```python
from build123d import *

# Parameters (mm, degrees)
SKETCH1_R           = 4.015
SKETCH1_R_2         = 3.015
BOSS_EXTRUDE1_DEPTH = 1.85
SKETCH2_R           = 4.05
BOSS_EXTRUDE2_DEPTH = 0.6
SKETCH3_R           = 2.05
SKETCH3_R_2         = 1.05
BOSS_EXTRUDE3_DEPTH = 6


with BuildPart() as part:
    # Sketch1 → Boss-Extrude1 (new body)
    with BuildSketch(Plane(origin=(0, 0, 0), x_dir=(1, 0, 0), z_dir=(0, 1, 0))):
        Circle(SKETCH1_R)
        Circle(SKETCH1_R_2, mode=Mode.SUBTRACT)
    extrude(amount=BOSS_EXTRUDE1_DEPTH)

    # Sketch2 → Boss-Extrude2 (add)
    with BuildSketch(Plane(origin=(0, 0, 0), x_dir=(1, 0, 0), z_dir=(0, 1, 0))):
        Circle(SKETCH2_R)
    extrude(amount=-BOSS_EXTRUDE2_DEPTH)

    # Sketch3 → Boss-Extrude3 (add)
    with BuildSketch(Plane.XZ.offset(0.6)):
        Circle(SKETCH3_R)
        Circle(SKETCH3_R_2, mode=Mode.SUBTRACT)
    extrude(amount=BOSS_EXTRUDE3_DEPTH)


solid = part.part
```
Here's how the part is built. I have some questions about the finished solid (model axes, mm). A direction names the side the tool comes from. Give positions to 0.01 mm unless a question says otherwise; leave off trailing zeros. Loops run counter-clockwise (first coordinate to the right, second up) from the corner with the lowest first, then second, coordinate; pieces in that order, holes last. Notation, with made-up numbers: M 83.25,84.5 L 114.25,84.5 A34 ccw 114.25,120.5 Z; hole C 38,25.5 d6. An arc over 180 degrees is marked long. Put each result on its own line as item: value. Start each with the question number.
(1) I want a section at C-C on y = 0.75. Please give me the cut outline in (x, z) (3 decimals), then the cut area to 3 significant figures.
(2) I need wall thicknesses on line 1 along Z through (x, y) = (0, 0.9) (3 decimals); line 2 along Z through (x, y) = (0, -2.25); line 3 along Y through (x, z) = (-1.5, 3.5). Which ranges of each line are inside material? Lowest first, please. Write a range as [from, to].
(3) I want a section at A-A on z = 0. Please give me the cut outline in (x, y) (3 decimals), then the cut area to 3 significant figures.
(4) Will these pins go through, and if not, where does the flat tip stop? pin 1 Ø3 at (x, z) = (1, -0.5) entering from +Y; pin 2 Ø1 at (x, z) = (3, -2.5) entering from -Y; pin 3 Ø3 at (x, y) = (-3, -5) entering from -Z; pin 4 Ø2.5 at (x, z) = (1, 0) entering from -Y.
(5) For faces 1 (the cylindrical face through (-0.654, 0.912, 2.943)), 2 (the flat face through (1, -6.6, -1)), 3 (the flat face through (-2, -0.6, -1)), which set-ups out of +Z, -Z, +X, -X, +Y, -Y let a thin tool reach every point of the face, with its end or its side?
(6) I want a section at B-B on x = 0. Please give me the cut outline in (y, z) (3 decimals).
(7) If we mould it in two halves opening along Z, with no side actions, what happens to faces 4 (the flat face through (-3, 1.85, -2)), 5 (the cylindrical face through (-0.878, -0.296, 3.954)), 6 (the flat face through (0, -0.6, 0))? For each: +Z half, -Z half, draft (parallel to the pull), parting line (faces both ways), or undercut.
Answer block:
1. outline: C 0,0 d8.03; hole C 0,0 d6.03
1. area: 22.1 mm^2
2. line 1: [-4.015, -3.015], [3.015, 4.015]
2. line 2: [-2.05, -1.05], [1.05, 2.05]
2. line 3: [-0.6, 1.85]
3. outline: M -4.05,-0.6 L -2.05,-0.6 L -2.05,-6.6 L -1.05,-6.6 L -1.05,-0.6 L 1.05,-0.6 L 1.05,-6.6 L 2.05,-6.6 L 2.05,-0.6 L 4.05,-0.6 L 4.05,0 L 4.015,0 L 4.015,1.85 L 3.015,1.85 L 3.015,0 L -3.015,0 L -3.015,1.85 L -4.015,1.85 L -4.015,0 L -4.05,0 Z
3. area: 20.6 mm^2
4. pin 1: y = 0
4. pin 2: y = -0.6
4. pin 3: z = -1.4
4. pin 4: y = -6.6
5. face 1: +Y
5. face 2: +Z, -Z, +X, -X, -Y
5. face 3: -Y
6. outline: M -6.6,-2.05 L -0.6,-2.05 L -0.6,-4.05 L 0,-4.05 L 0,-4.015 L 1.85,-4.015 L 1.85,-3.015 L 0,-3.015 L 0,3.015 L 1.85,3.015 L 1.85,4.015 L 0,4.015 L 0,4.05 L -0.6,4.05 L -0.6,2.05 L -6.6,2.05 L -6.6,1.05 L -0.6,1.05 L -0.6,-1.05 L -6.6,-1.05 Z
7. face 4: draft
7. face 5: parting line
7. face 6: undercut
